The listing builds one solid part. Answer for the finished solid, in the listing's coordinates (mm). Face numbers are marked on the shaded views. A direction names the side the tool comes from. Give positions to 0.01 mm unless a question says otherwise; leave off trailing zeros. Loops run counter-clockwise (first coordinate to the right, second up) from the corner with the lowest first, then second, coordinate; pieces in that order, holes last. Notation, with made-up numbers: (-6.5, -28.5) - (37.5, -28.5) arc R5 cw to (37.5, -22.5) - close; hole circle Ø8 at (-28, 14). An arc over 180 degrees is marked (long way). Answer as CSV lines item,"result". Start each with the question number.
1) A cutting plane is placed at D-D (x = 13.9). Determine the outline of the cut face in (y, z).
2) A cutting plane is placed at C-C (z = 7.5). Determine the outline of the cut face in (x, y), and give its area (3 significant figures).
3) A cutting plane is placed at A-A (x = 7.5). Give the number of separate pieces and of enclosed holes in the cut face, and give its area (3 significant figures).
4) Find the intervals of material crossed by line 1 along Y through (x, z) = (18.25, 11.5); line 2 along Y through (x, z) = (7.5, -1.8); line 3 along Y through (x, z) = (10.5, 4.5), in increasing order.
5) For a pull along Y with two mould halves and no side action, classify the marked faces 5, 6 and 7 as pulls with the +Y half, pulls with the -Y half, needs draft (parallel to the pull), parting line crosses it, or undercut.
6) For the marked faces 1, 2, 3 and 4, determine the directions among +Z, -Z, +X, -X, +Y, -Y from which every point of the face is accessible in a straight line to the end or side of a thin tool.
7) A cutting plane is placed at B-B (z = 10.75). Determine the outline of the cut face in (x, y).
8) Flat-ended cylindrical pins translate along their axes: pin 1 (3 mm diameter, centred on x = 10, y = 28.29, fed in from +Z); pin 2 (4 mm diameter, centred on x = 0, y = 33.29, fed in from +Z); pin 3 (2 mm diameter, centred on y = 40, z = -1.5, fed in from -X); pin 4 (4 mm diameter, centred on x = 14.5, z = 0.5, fed in from +Y). Find the tip coordinate at first contact, or state that the pin passes through.
```python
from build123d import *

# Parameters (mm, degrees)
SKETCH1_W           = 40
SKETCH1_H           = 50
SKETCH1_R           = 1.25
BASE_FLANGE1_DEPTH  = 2.5
SKETCH15_R          = 1
CUT_EXTRUDE3_DEPTH  = 10
JOG3_START          = -2.5
JOG3_OUTLINE_W      = 40
JOG3_OUTLINE_H      = 48.294687966
JOG3_OUTLINE_R      = 1
JOG3_OUTLINE_R_2    = 1.25
JOG3_DEPTH          = 2.5
JOG3_2_OUTLINE_W    = 40
JOG3_2_OUTLINE_H    = 1.705312034
JOG3_2_DEPTH        = 0.332528284
JOG3_START_2        = 14.2634
JOG3_3_OUTLINE_W    = 40
JOG3_3_OUTLINE_H    = 35
JOG3_3_OUTLINE_R    = 1
JOG3_3_OUTLINE_R_2  = 1.25
JOG3_3_DEPTH        = 3.2366
JOG3_4_OUTLINE_W    = 40
JOG3_4_OUTLINE_H    = 15.794687966
JOG3_4_OUTLINE_R    = 1.25
JOG3_4_DEPTH        = 3.2366
JOG3_5_OUTLINE_W    = 40
JOG3_5_OUTLINE_H    = 2.5
JOG3_5_DEPTH        = 15
JOG3_START_3        = 15
JOG3_6_OUTLINE_R    = 1.25
JOG3_6_OUTLINE_R_2  = 1
JOG3_6_DEPTH        = 2.5
JOG3_START_4        = -20
JOG3_7_DEPTH        = 40
JOG4_START          = -20
JOG4_DEPTH          = 40
JOG4_2_DEPTH        = 40
JOG4_START_2        = -3
JOG4_3_OUTLINE_R    = 1.25
JOG4_3_DEPTH        = 4
FILLET1_R           = 10
SKETCH18_R          = 2.5
BOSS_EXTRUDE1_DEPTH = 2.5
SKETCH19_R          = 1
SKETCH19_W          = 23.5
SKETCH19_H          = 12.5
CUT_EXTRUDE4_DEPTH  = 2.5
SKETCH20_R          = 2.5
SKETCH20_R_2        = 1.25
CUT_EXTRUDE6_DEPTH  = 10
SKETCH23_R          = 2.5
CUT_EXTRUDE7_DEPTH  = 44.945989578
SKETCH24_R          = 5
CUT_EXTRUDE8_DEPTH  = 1.25
SKETCH25_W          = 20
SKETCH25_H          = 13.5268
CUT_EXTRUDE11_DEPTH = 50.640775238


with BuildPart() as part:
    # Base-Flange1: sheet metal written as solids
    # Sketch1 → Base-Flange1 (new body)
    with BuildSketch(Plane.XY):
        Rectangle(SKETCH1_W, SKETCH1_H)
        with Locations((10, 12.5)):
            Circle(SKETCH1_R, mode=Mode.SUBTRACT)
        with Locations(Location((10, -12.5, 0), (0, 0, 180))):
            Circle(SKETCH1_R, mode=Mode.SUBTRACT)
        with Locations((-10, -12.5)):
            Circle(SKETCH1_R, mode=Mode.SUBTRACT)
        with Locations(Location((-10, 12.5, 0), (0, 0, 180))):
            Circle(SKETCH1_R, mode=Mode.SUBTRACT)
    extrude(amount=-BASE_FLANGE1_DEPTH)

    # Sketch15 → Cut-Extrude3 (cut)
    with BuildSketch(Plane.XY):
        with Locations((12, 0)):
            Circle(SKETCH15_R)
        with Locations(Location((-17, 0, 0), (0, 0, 180))):
            Circle(SKETCH15_R)
    extrude(amount=-CUT_EXTRUDE3_DEPTH, mode=Mode.SUBTRACT)

    # Jog3: read off the stored shape, not the designer's step
    # Jog3 outline → Jog3 (cut)
    with BuildSketch(Plane.XY.offset(JOG3_START)):
        with Locations((0, -0.852656017)):
            Rectangle(JOG3_OUTLINE_W, JOG3_OUTLINE_H)
        with Locations((-17, 0)):
            Circle(JOG3_OUTLINE_R, mode=Mode.SUBTRACT)
        with Locations((12, 0)):
            Circle(JOG3_OUTLINE_R, mode=Mode.SUBTRACT)
        with Locations((-10, 12.5)):
            Circle(JOG3_OUTLINE_R_2, mode=Mode.SUBTRACT)
        with Locations((10, 12.5)):
            Circle(JOG3_OUTLINE_R_2, mode=Mode.SUBTRACT)
        with Locations((10, -12.5)):
            Circle(JOG3_OUTLINE_R_2, mode=Mode.SUBTRACT)
        with Locations((-10, -12.5)):
            Circle(JOG3_OUTLINE_R_2, mode=Mode.SUBTRACT)
    extrude(amount=JOG3_DEPTH, mode=Mode.SUBTRACT)

    # Jog3 2 outline → Jog3 2 (cut)
    with BuildSketch(Plane.XY.offset(JOG3_START)):
        with Locations((0, 24.147343983)):
            Rectangle(JOG3_2_OUTLINE_W, JOG3_2_OUTLINE_H)
    extrude(amount=JOG3_2_DEPTH, mode=Mode.SUBTRACT)

    # Jog3 4 outline → Jog3 4 (add)
    with BuildSketch(Plane.XY.offset(JOG3_START)):
        with Locations((0, 32.897343983)):
            Rectangle(JOG3_4_OUTLINE_W, JOG3_4_OUTLINE_H)
        with Locations((10, 28.294687966)):
            Circle(JOG3_4_OUTLINE_R, mode=Mode.SUBTRACT)
        with Locations((-10, 28.294687966)):
            Circle(JOG3_4_OUTLINE_R, mode=Mode.SUBTRACT)
    extrude(amount=JOG3_4_DEPTH)



with BuildPart() as body_2:
    # Jog3 3 outline → Jog3 3 (new body)
    with BuildSketch(Plane.XY.offset(JOG3_START_2)):
        with Locations((0, 8.294687966)):
            Rectangle(JOG3_3_OUTLINE_W, JOG3_3_OUTLINE_H)
        with Locations((12, 15.794687966)):
            Circle(JOG3_3_OUTLINE_R, mode=Mode.SUBTRACT)
        with Locations((-17, 0)):
            Circle(JOG3_3_OUTLINE_R, mode=Mode.SUBTRACT)
        with Locations((-10, 3.294687966)):
            Circle(JOG3_3_OUTLINE_R_2, mode=Mode.SUBTRACT)
        with Locations((12, 0)):
            Circle(JOG3_3_OUTLINE_R, mode=Mode.SUBTRACT)
        with Locations((10, 3.294687966)):
            Circle(JOG3_3_OUTLINE_R_2, mode=Mode.SUBTRACT)
        with Locations((-17, 15.794687966)):
            Circle(JOG3_3_OUTLINE_R, mode=Mode.SUBTRACT)
        with Locations((-10, 12.5)):
            Circle(JOG3_3_OUTLINE_R_2, mode=Mode.SUBTRACT)
        with Locations((10, 12.5)):
            Circle(JOG3_3_OUTLINE_R_2, mode=Mode.SUBTRACT)
    extrude(amount=JOG3_3_DEPTH)


with BuildPart() as part_1:
    add(part.part)

    add(body_2.part)  # Jog3 5 merges body 2
    # Jog3 5 outline → Jog3 5 (add)
    with BuildSketch(Plane.XY):
        with Locations((0, 24.544687966)):
            Rectangle(JOG3_5_OUTLINE_W, JOG3_5_OUTLINE_H)
    extrude(amount=JOG3_5_DEPTH)

    # Jog3 6 outline → Jog3 6 (add)
    with BuildSketch(Plane.XY.offset(JOG3_START_3)):
        with Locations((10, 12.5)):
            Circle(JOG3_6_OUTLINE_R)
        with Locations((-10, 12.5)):
            Circle(JOG3_6_OUTLINE_R)
        with Locations((12, 0)):
            Circle(JOG3_6_OUTLINE_R_2)
        with Locations((-17, 0)):
            Circle(JOG3_6_OUTLINE_R_2)
    extrude(amount=JOG3_6_DEPTH)

    # Jog3 7 outline → Jog3 7 (cut)
    with BuildSketch(Plane.YZ.offset(JOG3_START_4)):
        with BuildLine():
            ThreePointArc((23.294687966, 14.2634), (23.078942821, 14.784254855), (22.558087966, 15))
            Line((22.558087966, 15), (-9.205312034, 15))
            Line((-9.205312034, 15), (-9.205312034, 14.2634))
            Line((-9.205312034, 14.2634), (23.294687966, 14.2634))
        make_face()
        with BuildLine():
            ThreePointArc((26.531287966, -2.5), (24.242666158, -1.552021808), (23.294687966, 0.7366))
            Line((23.294687966, 0.7366), (23.294687966, -2.167471716))
            Line((23.294687966, -2.167471716), (25, -2.167471716))
            Line((25, -2.167471716), (25, -2.5))
            Line((25, -2.5), (26.531287966, -2.5))
        make_face()
        with BuildLine():
            Line((26.531287966, 0), (40.794687966, 0))
            Line((40.794687966, 0), (40.794687966, 0.7366))
            Line((40.794687966, 0.7366), (25.794687966, 0.7366))
            ThreePointArc((25.794687966, 0.7366), (26.010433111, 0.215745145), (26.531287966, 0))
        make_face()
        with BuildLine():
            Line((25.794687966, 17.5), (22.558087966, 17.5))
            ThreePointArc((22.558087966, 17.5), (24.846709774, 16.552021808), (25.794687966, 14.2634))
            Line((25.794687966, 14.2634), (25.794687966, 17.5))
        make_face()
    extrude(amount=JOG3_7_DEPTH, mode=Mode.SUBTRACT)

    # Jog4: read off the stored shape, not the designer's step
    # Jog4 outline → Jog4 (cut)
    with BuildSketch(Plane.YZ.offset(JOG4_START)):
        with BuildLine():
            Line((-9.205312034, 15), (5.87962174, 15))
            ThreePointArc((5.87962174, 15), (7.019882984, 16.799110859), (9.031287966, 17.5))
            Line((9.031287966, 17.5), (-9.205312034, 17.5))
            Line((-9.205312034, 17.5), (-9.205312034, 15))
        make_face()
    extrude(amount=JOG4_DEPTH, mode=Mode.SUBTRACT)

    # Jog4 2 outline → Jog4 2 (add)
    with BuildSketch(Plane.YZ.offset(JOG4_START)):
        with BuildLine():
            Line((-9.205312034, 0), (-9.205312034, -2.5))
            Line((-9.205312034, -2.5), (5.058087966, -2.5))
            ThreePointArc((5.058087966, -2.5), (7.346709774, -1.552021808), (8.294687966, 0.7366))
            Line((8.294687966, 0.7366), (8.294687966, 14.2634))
            ThreePointArc((8.294687966, 14.2634), (8.510433111, 14.784254855), (9.031287966, 15))
            Line((9.031287966, 15), (5.87962174, 15))
            ThreePointArc((5.87962174, 15), (5.81599152, 14.634140241), (5.794687966, 14.2634))
            Line((5.794687966, 14.2634), (5.794687966, 0.7366))
            ThreePointArc((5.794687966, 0.7366), (5.578942821, 0.215745145), (5.058087966, 0))
            Line((5.058087966, 0), (-9.205312034, 0))
        make_face()
    extrude(amount=JOG4_2_DEPTH)

    # Jog4 3 outline → Jog4 3 (cut)
    with BuildSketch(Plane.XY.offset(JOG4_START_2)):
        with Locations((-10, 3.294687966)):
            Circle(JOG4_3_OUTLINE_R)
        with Locations((10, 3.294687966)):
            Circle(JOG4_3_OUTLINE_R)
    extrude(amount=JOG4_3_DEPTH, mode=Mode.SUBTRACT)

    # Fillet1
    fillet1_edges = [part_1.edges().sort_by_distance(p)[0] for p in [
        (20, -9.205312034, -1.25),
        (-20, -9.205312034, -1.25),
        (-20, 40.794687966, -1.25),
        (20, 40.794687966, -1.25),
    ]]
    fillet(fillet1_edges, radius=FILLET1_R)

    # Sketch18 → Boss-Extrude1 (add)
    with BuildSketch(Plane.XY.offset(17.5)):
        with Locations((12, 15.794687966)):
            Circle(SKETCH18_R)
        with Locations((-17, 15.794687966)):
            Circle(SKETCH18_R)
    extrude(amount=-BOSS_EXTRUDE1_DEPTH)

    # Sketch19 → Cut-Extrude4 (cut)
    with BuildSketch(Plane(origin=(0, 25.794687966, 0), x_dir=(1, 0, 0), z_dir=(0, 1, 0))):
        with Locations(Location((13.9, -7.5, 0), (0, 0, 270))):
            Circle(SKETCH19_R)
        with Locations(Location((-13.9, -7.5, 0), (0, 0, 90))):
            Circle(SKETCH19_R)
        with Locations((0, -7.5)):
            Rectangle(SKETCH19_W, SKETCH19_H)
    extrude(amount=-CUT_EXTRUDE4_DEPTH, mode=Mode.SUBTRACT)

    # Sketch20 → Cut-Extrude6 (cut)
    with BuildSketch(Plane.XY):
        with Locations((0, 33.294687966)):
            Circle(SKETCH20_R)
        with Locations(Location((0, -1.705312034, 0), (0, 0, 180))):
            Circle(SKETCH20_R)
        with Locations((7.5, -1.705312034)):
            Circle(SKETCH20_R_2)
        with Locations(Location((-7.5, -1.705312034, 0), (0, 0, 180))):
            Circle(SKETCH20_R_2)
        with Locations(Location((7.5, 33.294687966, 0), (0, 0, 180))):
            Circle(SKETCH20_R_2)
        with Locations((-7.5, 33.294687966)):
            Circle(SKETCH20_R_2)
    extrude(amount=-CUT_EXTRUDE6_DEPTH, mode=Mode.SUBTRACT)

    # Sketch23 → Cut-Extrude7 (cut, through all)
    with BuildSketch(Plane(origin=(0, 25.794687966, 0), x_dir=(1, 0, 0), z_dir=(0, 1, 0))):
        with Locations(Location((-5.55, -7.5, 0), (0, 0, 270))):
            Circle(SKETCH23_R)
    extrude(amount=-CUT_EXTRUDE7_DEPTH, mode=Mode.SUBTRACT)

    # Sketch24 → Cut-Extrude8 (cut)
    with BuildSketch(Plane(origin=(0, 8.294687966, 0), x_dir=(1, 0, 0), z_dir=(0, 1, 0))):
        with Locations(Location((-5.55, -7.5, 0), (0, 0, 270))):
            Circle(SKETCH24_R)
    extrude(amount=-CUT_EXTRUDE8_DEPTH, mode=Mode.SUBTRACT)

    # Sketch25 → Cut-Extrude11 (cut, through all)
    with BuildSketch(Plane.XY.offset(17.5)):
        Polygon((0, 38.294687966), (0, 40.794687966), (-20, 40.794687966), (-20, 22.558087966), (0, 22.558087966), (0, 28.294687966), (-5, 28.294687966), (-5, 38.294687966), align=None)
        with Locations((-10, 15.794687966)):
            Rectangle(SKETCH25_W, SKETCH25_H)
        Polygon((0, 9.031287966), (-20, 9.031287966), (-20, -9.205312034), (0, -9.205312034), (0, -6.705312034), (5, -6.705312034), (5, 3.294687966), (0, 3.294687966), align=None)
    extrude(amount=-CUT_EXTRUDE11_DEPTH, mode=Mode.SUBTRACT)


solid = part_1.part
```
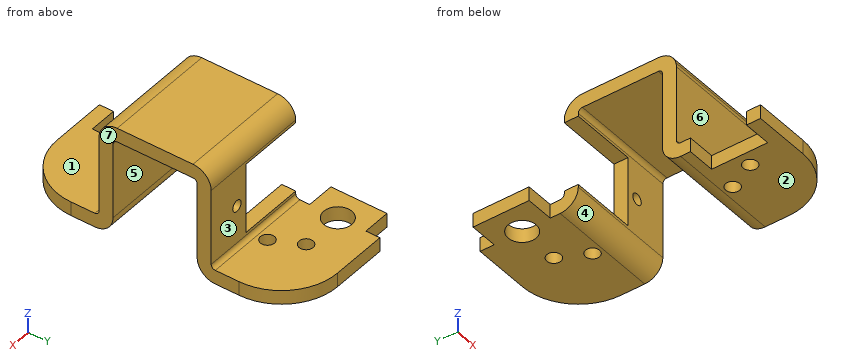
Ans:
1,outline,"(-8.41, -2.5) - (5.06, -2.5) arc R3.24 ccw to (8.29, 0.74) - (8.29, 14.26) arc R0.74 cw to (9.03, 15) - (22.56, 15) arc R0.74 cw to (23.29, 14.26) - (23.29, 8.5) - (25.79, 8.5) - (25.79, 14.26) arc R3.24 ccw to (22.56, 17.5) - (9.03, 17.5) arc R3.24 ccw to (5.79, 14.26) - (5.79, 0.74) arc R0.74 cw to (5.06, 0) - (-8.41, 0) - close; (23.29, 0.74) arc R3.24 ccw to (26.53, -2.5) - (40, -2.5) - (40, 0) - (26.53, 0) arc R0.74 cw to (25.79, 0.74) - (25.79, 6.5) - (23.29, 6.5) - close"
2,outline,"(0, 5.79) - (20, 5.79) - (20, 8.29) - (0, 8.29) - close; (11.75, 23.29) - (12.9, 23.29) - (12.9, 25.79) - (11.75, 25.79) - close; (14.9, 23.29) - (20, 23.29) - (20, 25.79) - (14.9, 25.79) - close"
2,area,"65.6 mm2"
3,separate pieces,"4"
3,enclosed holes,"0"
3,area,"160 mm2"
4,line 1,"5.79 to 8.29, 23.29 to 25.79"
4,line 2,"-9.21 to -2.96, -0.46 to 7.07, 24.52 to 32.04, 34.54 to 40.79"
4,line 3,"5.79 to 8.29"
5,face 5,"undercut"
5,face 6,"pulls with the -Y half"
5,face 7,"needs draft"
6,face 1,"+Z, +X, -X, -Y"
6,face 2,"-Z, +X, -X, +Y, -Y"
6,face 3,"+Z, +X, -X, +Y"
6,face 4,"-Z, +X, -X"
7,outline,"(0, 5.79) - (20, 5.79) - (20, 8.29) - (0, 8.29) - close; (11.75, 23.29) - (20, 23.29) - (20, 25.79) - (11.75, 25.79) - close"
8,pin 1,"z = 0"
8,pin 2,"through"
8,pin 3,"x = 0"
8,pin 4,"y = 40.46"
